Autodesk Inventor part; units mm, degrees
ref_plane "YZ Plane" through (0, 0, 0) normal (1, 0, 0) x (0, 1, 0)
ref_plane "XZ Plane" through (0, 0, 0) normal (0, 1, 0) x (-1, 0, 0)
ref_plane "XY Plane" through (0, 0, 0) normal (0, 0, 1) x (1, 0, 0)
sketch "Sketch1" plane through (0, 0, 0) normal (0, 0, 1) x (1, 0, 0)
  circle A0 centre (-21, 1.215) radius 1.4
  circle A1 centre (21, 1.215) radius 1.4
  arc A2 (24.9, 3.115) -> (22.9, 5.115) centre (22.9, 3.115) ccw
  line L0 (22.9, 5.115) -> (-22.9, 5.115)
  arc A3 (-22.9, 5.115) -> (-24.9, 3.115) centre (-22.9, 3.115) ccw
  line L1 (-24.9, 3.115) -> (-24.9, -5.115)
  line L2 (-24.9, -5.115) -> (24.9, -5.115)
  line L3 (24.9, -5.115) -> (24.9, 3.115)
  arc A4 (22.9, -44.685) -> (24.9, -42.685) centre (22.9, -42.685) ccw
  line L4 (24.9, -42.685) -> (24.9, -36.885)
  line L5 (24.9, -36.885) -> (17.1, -36.885)
  line L6 (17.1, -36.885) -> (17.1, -44.685)
  line L7 (17.1, -44.685) -> (22.9, -44.685)
  circle A5 centre (21, -40.785) radius 1.4
  arc A6 (-24.9, -42.685) -> (-22.9, -44.685) centre (-22.9, -42.685) ccw
  line L8 (-22.9, -44.685) -> (-17.1, -44.685)
  line L9 (-17.1, -44.685) -> (-17.1, -36.885)
  line L10 (-17.1, -36.885) -> (-24.9, -36.885)
  line L11 (-24.9, -36.885) -> (-24.9, -42.685)
  circle A7 centre (-21, -40.785) radius 1.4
  line L12 (24.9, 5.115) -> (-24.9, 5.115)
  line L13 (-24.9, 5.115) -> (-24.9, -44.685)
  line L14 (-24.9, -44.685) -> (24.9, -44.685)
  line L15 (24.9, -44.685) -> (24.9, 5.115)
  line L16 (17.1, -2.685) -> (-17.1, -2.685)
  line L17 (-17.1, -2.685) -> (-17.1, -36.885)
  line L18 (-17.1, -36.885) -> (17.1, -36.885)
  line L19 (17.1, -36.885) -> (17.1, -2.685)
  line L20 (17.1, -36.885) -> (17.1, -44.685)
  line L21 (-17.1, -36.885) -> (-17.1, -44.685)
  circle A8 centre (0, 1.415) radius 1.4
  point P0 (0, 0)
  dimension "d0" = 7.8
extrude "Extrusion1" add sketch "Sketch1" along normal blind 8 contours L3 L2 L19 L16 L17 L1 A3 L0 A2 | L15 L5 L19 L2 | L4 A4 L7 L6 L5 | L17 L10 L13 L2 | L9 L8 A6 L11 L10 | A8
sketch "Sketch2" plane through (0, 0, 8) normal (0, 0, 1) x (1, 0, 0)
  circle A0 centre (0, 1.715) radius 1.4
  line L0 (22.9, 5.115) -> (-22.9, 5.115)
  point P0 (0, 0)
  dimension "d3" = 2.8
  dimension "d4" = 3.4
extrude "Extrusion2" cut sketch "Sketch2" against normal blind 8
properties part number "00_Linear_Stage_NEMA11_Mount_Lid"
Read the model definition and answer for the solid it produces. Units are mm, in the model's axes. A direction names the side the tool comes from. Coordinates: 2 decimals unless noted, no trailing zeros. Order: outer loops, then holes, each group sorted by start corner. A loop starts at its lowest first (then second) coordinate and runs counter-clockwise, first axis right, second up. Notation, with made-up numbers: (81.5, -33) - (101.5, -33) arc R9 cw to (101.5, -26) - close; hole circle Ø4 at (69.5, 80). An arc over 180 degrees is marked (long way). Answer as a JSON object with one key per item and string values. Group by question number.
Item 1: The mould has two halves that part along Y. Classify faces 3 (the face through (0, -2.685, 4)), 4 (the face through (24.299, 4.545, 3.944)), 5 (the face through (-24.9, -19, 4)), 6 (the face through (22.293, -40.249, 3.944)): +Y half, -Y half, draft (parallel to the pull), parting line (faces both ways), or undercut.
Item 2: Section C-C (y = -35) is taken. Give the vertices of the cut face in (x, z), plus the area to 3 significant figures.
Item 3: Section A-A (x = 0) is taken. Give the vertices of the cut face in (y, z) (3 decimals).
Item 4: Section D-D (z = 4.5) is taken. Give the vertices of the cut face in (x, y) (3 decimals), plus the area to 3 significant figures.
Item 5: Section B-B (x = 21) is taken. Give the vertices of the cut face in (y, z) (3 decimals), plus the area to 3 significant figures.
Item 6: Consider probe 1 along Y at (x, z) = (-21, 4) (3 decimals); probe 2 along X at (y, z) = (-25, 6.25); probe 3 along X at (y, z) = (1, 4.75). Determine where each line is inside the solid, lowest interval first. Write a range as from..to.
Item 7: A tool of negligible diameter and unlimited length cuts with its end or side. For faces 1 (the face through (17.1, -24, 4)), 2 (the face through (-20, -44.685, 4)), from which of +Z, -Z, +X, -X, +Y, -Y can it reach the whole face along a straight path? Write none if from no direction.
Item 8: Flat-ended cylindrical pins translate along their axes: P1, Ø1.7, axis at x = 0, y = 1.715, coming from the -Z side; P2, Ø3.5, axis at x = 21, y = 1.215, coming from the -Z side; P3, Ø2.5, axis at x = 4, z = 3.5, coming from the -Y side (3 decimals). Find the tip coordinate at first contact, or state that the pin passes through.
Results are:
{
 "1": {"face 3": "-Y half", "face 4": "+Y half", "face 5": "draft", "face 6": "undercut"},
 "2": {"outline": "(-24.9, 0) - (-17.1, 0) - (-17.1, 8) - (-24.9, 8) - close; (17.1, 0) - (24.9, 0) - (24.9, 8) - (17.1, 8) - close", "area": "125 mm^2"},
 "3": {"outline": "(-2.685, 0) - (0.315, 0) - (0.315, 8) - (-2.685, 8) - close; (3.115, 0) - (5.115, 0) - (5.115, 8) - (3.115, 8) - close"},
 "4": {"outline": "(-24.9, -42.685) arc R2 ccw to (-22.9, -44.685) - (-17.1, -44.685) - (-17.1, -2.685) - (17.1, -2.685) - (17.1, -44.685) - (22.9, -44.685) arc R2 ccw to (24.9, -42.685) - (24.9, 3.115) arc R2 ccw to (22.9, 5.115) - (-22.9, 5.115) arc R2 ccw to (-24.9, 3.115) - close; hole circle Ø2.8 at (-21, -40.785); hole circle Ø2.8 at (-21, 1.215); hole circle Ø2.8 at (0, 1.715); hole circle Ø2.8 at (21, -40.785); hole circle Ø2.8 at (21, 1.215)", "area": "1,010 mm^2"},
 "5": {"outline": "(-44.685, 0) - (-42.185, 0) - (-42.185, 8) - (-44.685, 8) - close; (-39.385, 0) - (-0.185, 0) - (-0.185, 8) - (-39.385, 8) - close; (2.615, 0) - (5.115, 0) - (5.115, 8) - (2.615, 8) - close", "area": "354 mm^2"},
 "6": {"probe 1": "y = -44.685..-42.185, -39.385..-0.185, 2.615..5.115", "probe 2": "x = -24.9..-17.1, 17.1..24.9", "probe 3": "x = -24.9..-22.38, -19.62..-1.2, 1.2..19.62, 22.38..24.9"},
 "7": {"face 1": "+Z, -Z, -Y", "face 2": "+Z, -Z, +X, -X, -Y"},
 "8": {"P1": "passes through", "P2": "stops at z = 0", "P3": "stops at y = -2.685"}
}
